Design review of the part built by this model. Coordinates are the model's own, in mm. Face numbers are marked on the shaded views. A direction names the side the tool comes from. Coordinates: 2 decimals unless noted, no trailing zeros. Loops run counter-clockwise (first coordinate to the right, second up) from the corner with the lowest first, then second, coordinate; pieces in that order, holes last. Notation, with made-up numbers: (18.25, 82.5) -> (72.25, 82.5) arc R18 cw to (72.25, 106.5) -> close; hole circle Ø10 at (12, 75.25). An arc over 180 degrees is marked (long way). Answer as a JSON object with one key per item and string values.
```python
from build123d import *

# Parameters (mm, degrees)
CROQUIS1_W              = 30
CROQUIS1_H              = 30
SALIENTE_EXTRUIR1_DEPTH = 3
CROQUIS2_W              = 9.563107214
CROQUIS2_H              = 25.610650669
SALIENTE_EXTRUIR2_DEPTH = 30
CROQUIS3_R              = 4.0394072
CORTAR_EXTRUIR1_DEPTH   = 10


with BuildPart() as part:
    # Croquis1 → Saliente-Extruir1 (new body)
    with BuildSketch(Plane(origin=(0, 0, 0), x_dir=(1, 0, 0), z_dir=(0, 1, 0))):
        Rectangle(CROQUIS1_W, CROQUIS1_H)
    extrude(amount=SALIENTE_EXTRUIR1_DEPTH)

    # Croquis2 → Saliente-Extruir2 (add)
    with BuildSketch(Plane(origin=(0, 3, 0), x_dir=(1, 0, 0), z_dir=(0, 1, 0))):
        with Locations((0.232305854, 2.194674666)):
            Rectangle(CROQUIS2_W, CROQUIS2_H)
    extrude(amount=SALIENTE_EXTRUIR2_DEPTH)

    # Croquis3 → Cortar-Extruir1 (cut)
    with BuildSketch(Plane(origin=(5.013859461, 0, 0), x_dir=(0, 0, -1), z_dir=(1, 0, 0))):
        with Locations((0.584677198, 25.603738422)):
            Circle(CROQUIS3_R)
    extrude(amount=-CORTAR_EXTRUIR1_DEPTH, mode=Mode.SUBTRACT)


solid = part.part
```
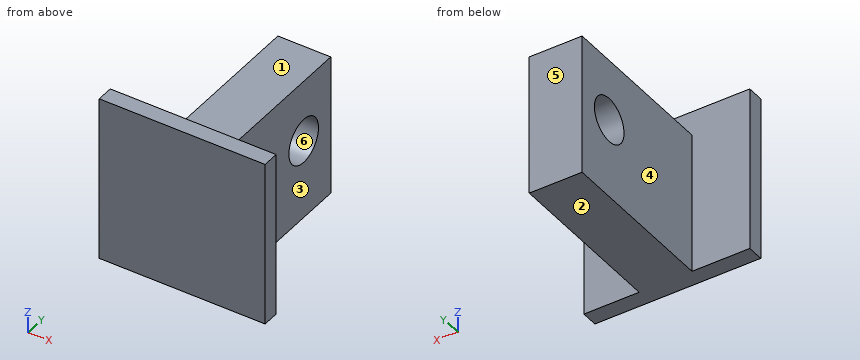
1) Add section C-C, the plane z = 9. Give the boundary of the cut face in (x, y).
Completed:
{"outline": "(-15, 0) -> (15, 0) -> (15, 3) -> (5.01, 3) -> (5.01, 33) -> (-4.55, 33) -> (-4.55, 3) -> (-15, 3) -> close"}
2) Add section D-D, the plane z = 2. Give the boundary of the cut face in (x, y).
Completed:
{"outline": "(-15, 0) -> (15, 0) -> (15, 3) -> (5.01, 3) -> (5.01, 22.5) -> (-4.55, 22.5) -> (-4.55, 3) -> (-15, 3) -> close; (-4.55, 28.71) -> (5.01, 28.71) -> (5.01, 33) -> (-4.55, 33) -> close"}
3) Wall thickness on probe 1 along X at (y, z) = (12.5, 3); probe 2 along Y at (x, z) = (-10.25, -6); probe 3 along Y at (x, z) = (-2.5, 0): over which ranges is each line inside the solid? List them lowest first.
Completed:
{"probe 1": "-4.55 to 5.01", "probe 2": "0 to 3", "probe 3": "0 to 21.61, 29.6 to 33"}
4) Add section A-A, the plane z = -3.5. Give the boundary of the cut face in (x, y), and give its area (3 significant figures).
Completed:
{"outline": "(-15, 0) -> (15, 0) -> (15, 3) -> (5.01, 3) -> (5.01, 22.81) -> (-4.55, 22.81) -> (-4.55, 3) -> (-15, 3) -> close; (-4.55, 28.4) -> (5.01, 28.4) -> (5.01, 33) -> (-4.55, 33) -> close", "area": "323 mm²"}
5) For the marked faces 1, 2 and 3, list the 3-axis set-ups (+Z, -Z, +X, -X, +Y, -Y) from which the entire face can be reached by the end or side of a thin tool; tool diameter is ignored.
Completed:
{"face 1": "+Z, +X, -X, +Y", "face 2": "-Z, +X, -X, +Y, -Y", "face 3": "+Z, -Z, +X, +Y"}
6) Clearance check with flat-ended pins moving along their axes: pin 1 Ø10.5 at (x, y) = (-2, 14.5) entering from +Z; pin 2 Ø1 at (x, z) = (-5.5, -3) entering from -Y; pin 3 Ø1 at (y, z) = (8, 1) entering from +X. State where each tip first meets the part, or that it passes through.
Completed:
{"pin 1": "z = 10.61", "pin 2": "y = 0", "pin 3": "x = 5.01"}
7) Add section B-B, the plane y = 25. Give the boundary of the cut face in (x, z), and give its area (3 significant figures).
Completed:
{"outline": "(-4.55, -15) -> (5.01, -15) -> (5.01, -4.58) -> (-4.55, -4.58) -> close; (-4.55, 3.41) -> (5.01, 3.41) -> (5.01, 10.61) -> (-4.55, 10.61) -> close", "area": "169 mm²"}
8) The part is to be moulded in two halves that separate along Y. For the marked faces 4, 5 and 6, say which applies: pulls with the +Y half, pulls with the -Y half, needs draft (parallel to the pull), parting line crosses it, or undercut.
Completed:
{"face 4": "needs draft", "face 5": "pulls with the +Y half", "face 6": "undercut"}
